Part model, mm, in its own coordinate system. A direction names the side the tool comes from. Give positions to 0.01 mm unless a question says otherwise; leave off trailing zeros. Write each loop counter-clockwise with the first axis right and the second up, starting at its lowest first coordinate (ties: lowest second). Pieces come first, ordered by that corner, then holes. Notation, with made-up numbers: (77.5, -13.5) - (95.5, -13.5) arc R12 cw to (95.5, 0.5) - close; hole circle Ø10 at (-16, -5). An arc over 180 degrees is marked (long way). Answer in a Markdown table with one row per item. Add a question column.
1. Probe line 1 along Z through (x, y) = (0, 101.85); line 2 along Y through (x, z) = (44.5, 1); line 3 along Z through (x, y) = (0, 80.4). List the from-to ranges inside material, lowest first.
2. Band-saw the part on A-A on z = 0. Write the cut outline in (x, y).
3. Band-saw the part on B-B on x = 0. State how many separate pieces and enclosed holes the cut face has, plus the area to 3 significant figures.
4. Band-saw the part on C-C on z = -46. Write the cut outline in (x, y), plus the area to 3 significant figures.
5. Pull direction Z, two halves, no side cores. Call faces 1 (the cylindrical face through (-18.49, 80.49, 14.67)), 2 (the cylindrical face through (0.976, 101.507, 72.436)), 3 (the flat face through (-18, 80, -1)), 4 (the cylindrical face through (-39.22, 101.49, 75.41)): released by +Z, released by -Z, zero draft, split by the parting line, or undercut.
6. Drop flat-ended pins along their axis: pin 1 Ø12 at (y, z) = (67, -1.5) entering from +X; pin 2 Ø1.5 at (x, z) = (-18.5, 31) entering from -Y; pin 3 Ø12 at (x, z) = (0, 30) entering from -Y; pin 4 Ø17 at (x, z) = (65, 0) entering from +Y. Give the stop position or say it passes through.
7. Which spindle directions (+Z, -Z, +X, -X, +Y, -Y) get a long thin tool onto all of the face, cutting with end or side? Do faces 5 (the cylindrical face through (31.51, 80.49, 9.93)), 6 (the cylindrical face through (32.17, 101.51, -48.8)), 7 (the cylindrical face through (-39.22, 80.49, 75.41)). Say none if no direction does.
8. Band-saw the part on D-D on x = -70. Write the cut outline in (y, z), plus the area to 3 significant figures.
```python
from build123d import *

# Parameters (mm, degrees)
SKETCH2_R          = 7.5
CUT_EXTRUDE1_DEPTH = 2
CIRPATTERN1_COUNT  = 12
SKETCH3_R          = 7.5
CUT_EXTRUDE2_DEPTH = 2
CIRPATTERN2_COUNT  = 6


with BuildPart() as part:
    # Sketch1 → Revolve1 (revolve)
    with BuildSketch(Plane.XY):
        Polygon((0, 102), (-84.99983, 102), (-84.99983, 101), (-5, 101), (-5, 81), (-84.99983, 81), (-84.99983, 80), (-5, 80), (-5, 0), (0, 0), align=None)
    revolve(axis=Axis((0, 54.874193188, 0), (0, -1, 0)))

    # Sketch2 → Cut-Extrude1 (cut)
    with BuildSketch(Plane(origin=(0, 102, 0), x_dir=(1, 0, 0), z_dir=(0, 1, 0))):
        with Locations((0, 65)):
            Circle(SKETCH2_R)
    cut_extrude1 = extrude(amount=-CUT_EXTRUDE1_DEPTH, mode=Mode.SUBTRACT)

    # CirPattern1: Cut-Extrude1 ×12 about axis
    cirpattern1_axis = Axis((0, 0, 0), (0, 1, 0))
    for i in range(1, CIRPATTERN1_COUNT):
        add(cut_extrude1.rotate(cirpattern1_axis, i * 360 / CIRPATTERN1_COUNT), mode=Mode.SUBTRACT)

    # Sketch3 → Cut-Extrude2 (cut)
    with BuildSketch(Plane.XZ.offset(-80)):
        with Locations((0, 30)):
            Circle(SKETCH3_R)
    cut_extrude2 = extrude(amount=-CUT_EXTRUDE2_DEPTH, mode=Mode.SUBTRACT)

    # CirPattern2: Cut-Extrude2 ×6 about axis
    cirpattern2_axis = Axis((0, 0, 0), (0, 1, 0))
    for i in range(1, CIRPATTERN2_COUNT):
        add(cut_extrude2.rotate(cirpattern2_axis, i * 360 / CIRPATTERN2_COUNT), mode=Mode.SUBTRACT)


solid = part.part
```
Values:
| question | item | result |
|---|---|---|
| 1 | line 1 | z = -85 to -72.5, -57.5 to 57.5, 72.5 to 85 |
| 1 | line 2 | y = 80 to 81, 101 to 102 |
| 1 | line 3 | z = -85 to -37.5, -22.5 to 22.5, 37.5 to 85 |
| 2 | outline | (-85, 80) - (-5, 80) - (-5, 0) - (5, 0) - (5, 80) - (85, 80) - (85, 81) - (5, 81) - (5, 101) - (57.5, 101) - (57.5, 102) - (-57.5, 102) - (-57.5, 101) - (-5, 101) - (-5, 81) - (-85, 81) - close; (-85, 101) - (-72.5, 101) - (-72.5, 102) - (-85, 102) - close; (72.5, 101) - (85, 101) - (85, 102) - (72.5, 102) - close |
| 3 | separate pieces | 5 |
| 3 | enclosed holes | 0 |
| 3 | area | 1,280 mm² |
| 4 | outline | (-71.48, 80) - (71.48, 80) - (71.48, 81) - (-71.48, 81) - close; (-71.48, 101) - (71.48, 101) - (71.48, 102) - (-71.48, 102) - close |
| 4 | area | 286 mm² |
| 5 | face 1 | undercut |
| 5 | face 2 | undercut |
| 5 | face 3 | zero draft |
| 5 | face 4 | split by the parting line |
| 6 | pin 1 | stops at x = 5 |
| 6 | pin 2 | stops at y = 80 |
| 6 | pin 3 | stops at y = 101 |
| 6 | pin 4 | stops at y = 102 |
| 7 | face 5 | -Y |
| 7 | face 6 | +Y |
| 7 | face 7 | +Y, -Y |
| 8 | outline | (80, -48.22) - (81, -48.22) - (81, 48.22) - (80, 48.22) - close; (101, -48.22) - (102, -48.22) - (102, -5.59) - (101, -5.59) - close; (101, 5.59) - (102, 5.59) - (102, 48.22) - (101, 48.22) - close |
| 8 | area | 182 mm² |
